Can you work these out from the model? Positions are in its coordinate system, mm. Coordinates: 2 decimals unless noted, no trailing zeros. Order: outer loops, then holes, each group sorted by start corner. A loop starts at its lowest first (then second) coordinate and runs counter-clockwise, first axis right, second up.
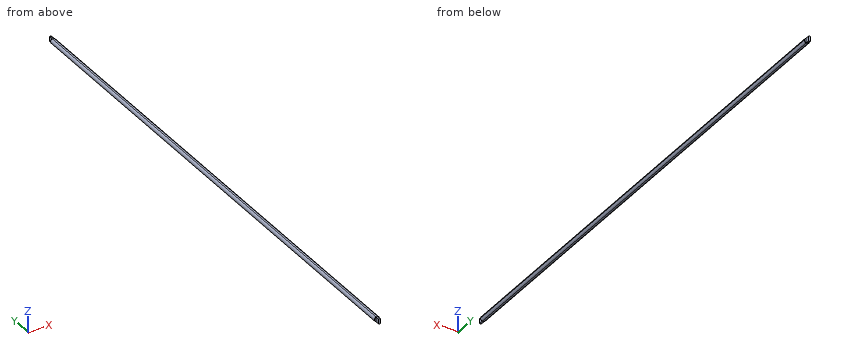
```python
from build123d import *

# Parameters (mm, degrees)
SKETCH1_R           = 3
BOSS_EXTRUDE1_DEPTH = 616.37
BOSS_EXTRUDE3_DEPTH = 5
SKETCH4_W           = 2
SKETCH4_H           = 5.65685425
BOSS_EXTRUDE4_DEPTH = 641.64
SKETCH5_W           = 2
SKETCH5_H           = 5.65685425
CUT_EXTRUDE2_DEPTH  = 15.27


with BuildPart() as part:
    # Sketch1 → Boss-Extrude1 (new body)
    with BuildSketch(Plane(origin=(0, 0, 0), x_dir=(1, 0, 0), z_dir=(0, 1, 0))):
        Circle(SKETCH1_R)
    extrude(amount=BOSS_EXTRUDE1_DEPTH)

    # Sketch2 → Boss-Extrude3 (add)
    with BuildSketch(Plane(origin=(0, 616.37, 0), x_dir=(1, 0, 0), z_dir=(0, 1, 0))):
        with BuildLine():
            ThreePointArc((-1, -2.828427125), (-0.507305936, -2.956795679), (0, -3))
            ThreePointArc((0, -3), (0.507305936, -2.956795679), (1, -2.828427125))
            Line((1, -2.828427125), (1, 2.828427125))
            ThreePointArc((1, 2.828427125), (0.507305936, 2.956795679), (0, 3))
            ThreePointArc((0, 3), (-0.507305936, 2.956795679), (-1, 2.828427125))
            Line((-1, 2.828427125), (-1, -2.828427125))
        make_face()
    extrude(amount=BOSS_EXTRUDE3_DEPTH)

    # Sketch4 → Boss-Extrude4 (add)
    with BuildSketch(Plane(origin=(0, 621.37, 0), x_dir=(1, 0, 0), z_dir=(0, 1, 0))):
        Rectangle(SKETCH4_W, SKETCH4_H)
        with BuildLine():
            Line((-1, -2.828427125), (1, -2.828427125))
            ThreePointArc((1, -2.828427125), (0, -3), (-1, -2.828427125))
        make_face()
        with BuildLine():
            Line((-1, 2.828427125), (1, 2.828427125))
            ThreePointArc((1, 2.828427125), (0, 3), (-1, 2.828427125))
        make_face()
    extrude(amount=-BOSS_EXTRUDE4_DEPTH)

    # Sketch5 → Cut-Extrude2 (cut)
    with BuildSketch(Plane.XZ.offset(20.27)):
        with BuildLine():
            Line((-1, -2.828427125), (1, -2.828427125))
            ThreePointArc((1, -2.828427125), (0, -3), (-1, -2.828427125))
        make_face()
        Rectangle(SKETCH5_W, SKETCH5_H)
        with BuildLine():
            Line((-1, 2.828427125), (1, 2.828427125))
            ThreePointArc((1, 2.828427125), (0, 3), (-1, 2.828427125))
        make_face()
    extrude(amount=-CUT_EXTRUDE2_DEPTH, mode=Mode.SUBTRACT)


solid = part.part
```
1. Imagine slicing it at B-B on y = 540. Please give me the cut outline in (x, z), then the cut area to 3 significant figures.
Completed:
outline: circle Ø6 at (0, 0)
area: 28.3 mm2
2. I'm going to push flat-ended pins straight in: pin 1 (1.6 mm diameter, centred on x = -2.5, z = 1, fed in from +Y); pin 2 (2.5 mm diameter, centred on y = 619.5, z = 1, fed in from +X); pin 3 (1 mm diameter, centred on x = -1, y = 390, fed in from +Z). Where does each tip first touch, or does it pass through?
Completed:
pin 1: stops at y = 616.37
pin 2: stops at x = 1
pin 3: stops at z = 2.96
3. Imagine slicing it at A-A on z = 1. Please give me the cut outline in (x, y).
Completed:
outline: (-2.83, 0) - (-1, 0) - (-1, -5) - (1, -5) - (1, 0) - (2.83, 0) - (2.83, 616.37) - (1, 616.37) - (1, 621.37) - (-1, 621.37) - (-1, 616.37) - (-2.83, 616.37) - close
4. Please list where these lines run through material, in increasing order: probe 1 along X at (y, z) = (592, 0.5); probe 2 along Y at (x, z) = (2.3, 0.75); probe 3 along X at (y, z) = (457.5, -0.75).
Completed:
probe 1: x = -2.96 to 2.96
probe 2: y = 0 to 616.37
probe 3: x = -2.9 to 2.9
5. Imagine slicing it at C-C on x = 2. Please give me the cut outline in (y, z), then the cut area to 3 significant figures.
Completed:
outline: (0, -2.24) - (616.37, -2.24) - (616.37, 2.24) - (0, 2.24) - close
area: 2,760 mm2
